```python
from build123d import *

# Parameters (mm, degrees)
F1_DEPTH = 75
F2_R     = 5


with BuildPart() as f1:
    # F0 (on Front) → F1 (new body, symmetric)
    with BuildSketch(Plane.XZ):
        Polygon((-71.73389, -43.765602), (-121.73389, -43.765602), (-121.73389, -93.765602), (178.26611, -93.765602), (178.26611, -43.765602), (128.26611, -43.765602), align=None)
        Polygon((-71.73389, 76.234398), (-71.73389, -43.765602), (128.26611, -43.765602), (128.26611, 76.234398), (53.26611, 76.234398), (53.26611, -23.765602), (3.26611, -23.765602), (3.26611, 76.234398), align=None)
    extrude(amount=F1_DEPTH, both=True)

    # F2
    f2_edges = [f1.edges().sort_by_distance(p)[0] for p in [
        (53.26611, 0, 76.234398),
        (3.26611, 0, 76.234398),
        (128.26611, 0, 76.234398),
        (-71.73389, 0, 76.234398),
        (-71.73389, 0, -43.765602),
        (-121.73389, 0, -43.765602),
        (128.26611, 0, -43.765602),
        (178.26611, 0, -43.765602),
        (3.26611, 0, -23.765602),
        (53.26611, 0, -23.765602),
    ]]
    fillet(f2_edges, radius=F2_R)


solid = f1.part
```
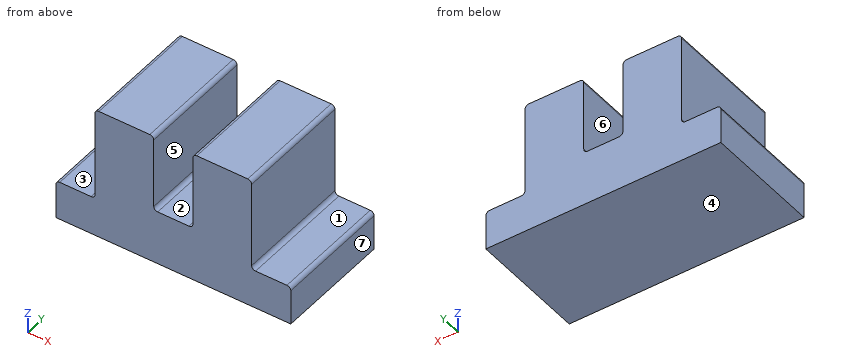
Can you work these out from the model? Positions are in its coordinate system, mm. Face numbers are marked on the shaded views. A direction names the side the tool comes from. Round coordinates to 2 decimals unless told otherwise and drop trailing zeros. Loops run counter-clockwise (first coordinate to the right, second up) from the corner with the lowest first, then second, coordinate; pieces in that order, holes last.
Item 1: Suppose I cut it at B-B, the plane y = 8.5. Write out the boundary of the cut face in (x, z), then the cut area to 3 significant figures.
Item 2: Suppose I cut it at A-A, the plane z = 42. Write out the boundary of the cut face in (x, y).
Item 3: Will these pins go through, and if not, where does the flat tip stop? pin 1 Ø5 at (y, z) = (41.5, 3.5) entering from +X; pin 2 Ø3 at (y, z) = (16, -2.5) entering from -X; pin 3 Ø20 at (x, y) = (-102.5, -23.5) entering from +Z.
Item 4: Suppose I cut it at D-D, the plane z = -28.5. Write out the boundary of the cut face in (x, y).
Item 5: Please list where these lines run through material, in increasing order: L1, parallel to X at y = 22.5, z = 31; L2, parallel to Z at x = 19.5, y = 12.5; L3, parallel to X at y = 30.5, z = -39.5.
Item 6: Which directions (+Z, -Z, +X, -X, +Y, -Y) give clear straight access to the entire face, cutting with the end or side of a thin tool? Please do the marked faces 1, 2 and 3.
Item 7: If we mould it in two halves opening along X, with no side actions, what happens to the marked faces 4, 5, 6 and 7? For each: +X half, -X half, draft (parallel to the pull), parting line (faces both ways), or undercut.
Item 8: Suppose I cut it at C-C, the plane x = 32. Write out the boundary of the cut face in (y, z).
Reported:
1. outline: (-121.73, -93.77) - (178.27, -93.77) - (178.27, -48.77) arc R5 ccw to (173.27, -43.77) - (133.27, -43.77) arc R5 cw to (128.27, -38.77) - (128.27, 71.23) arc R5 ccw to (123.27, 76.23) - (58.27, 76.23) arc R5 ccw to (53.27, 71.23) - (53.27, -18.77) arc R5 cw to (48.27, -23.77) - (8.27, -23.77) arc R5 cw to (3.27, -18.77) - (3.27, 71.23) arc R5 ccw to (-1.73, 76.23) - (-66.73, 76.23) arc R5 ccw to (-71.73, 71.23) - (-71.73, -38.77) arc R5 cw to (-76.73, -43.77) - (-116.73, -43.77) arc R5 ccw to (-121.73, -48.77) - close
1. area: 34,000 mm2
2. outline: (-71.73, -75) - (3.27, -75) - (3.27, 75) - (-71.73, 75) - close; (53.27, -75) - (128.27, -75) - (128.27, 75) - (53.27, 75) - close
3. pin 1: stops at x = 128.27
3. pin 2: stops at x = -71.73
3. pin 3: stops at z = -43.77
4. outline: (-71.73, -75) - (128.27, -75) - (128.27, 75) - (-71.73, 75) - close
5. L1: x = -71.73 to 3.27, 53.27 to 128.27
5. L2: z = -93.77 to -23.77
5. L3: x = -71.79 to 128.32
6. face 1: +Z, +X, +Y, -Y
6. face 2: +Z, +Y, -Y
6. face 3: +Z, -X, +Y, -Y
7. face 4: draft
7. face 5: undercut
7. face 6: undercut
7. face 7: +X half
8. outline: (-75, -93.77) - (75, -93.77) - (75, -23.77) - (-75, -23.77) - close
